Here's the drawing with two shaded views (mm, measured from the low corner). I have some questions. Coordinates: 2 decimals unless noted, no trailing zeros. Loops run counter-clockwise (first coordinate to the right, second up) from the corner with the lowest first, then second, coordinate; pieces in that order, holes last.
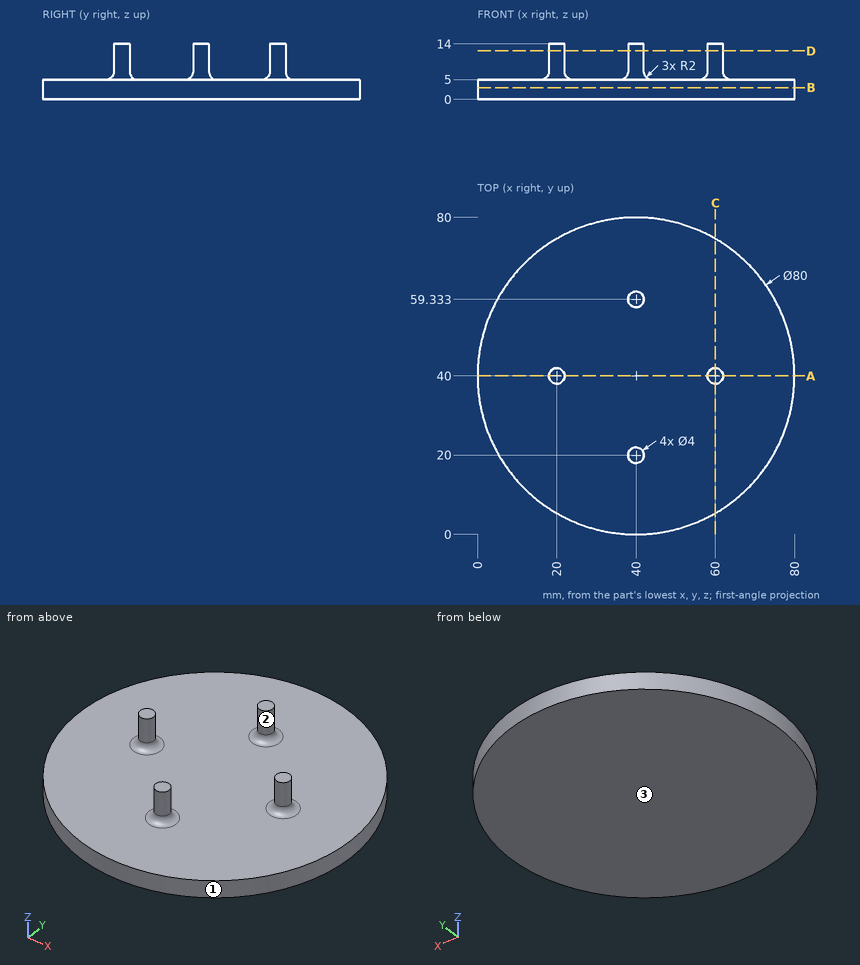
(1) I'm going to push flat-ended pins straight in: pin 1 (4 mm diameter, centred on x = 65.5, y = 39, fed in from -Z); pin 2 (5 mm diameter, centred on x = 53, y = 18, fed in from +Z); pin 3 (6 mm diameter, centred on y = 36, z = 2, fed in from -X); pin 4 (2 mm diameter, centred on x = 32.5, z = 4, fed in from -Y). Where does each tip first touch, or does it pass through?
Check values:
pin 1: stops at z = 0
pin 2: stops at z = 5
pin 3: stops at x = 0.01
pin 4: stops at y = 0.53
(2) If we mould it in two halves opening along Y, with no side actions, what happens to the marked faces 1, 2 and 3? For each: released by +Y, released by -Y, zero draft, split by the parting line, or undercut.
Check values:
face 1: split by the parting line
face 2: undercut
face 3: zero draft
(3) I want a section at A-A on y = 40. Write out the boundary of the cut face in (x, z).
Check values:
outline: (0, 0) - (80, 0) - (80, 5) - (64, 5) arc R2 cw to (62, 7) - (62, 14) - (58, 14) - (58, 7) arc R2 cw to (56, 5) - (24, 5) arc R2 cw to (22, 7) - (22, 14) - (18, 14) - (18, 7) arc R2 cw to (16, 5) - (0, 5) - close
(4) I want a section at B-B on z = 3. Write out the boundary of the cut face in (x, y), then the cut area to 3 significant figures.
Check values:
outline: circle Ø80 at (40, 40)
area: 5,030 mm2
(5) If I drill on probe 1 along Z at (x, y) = (26, 76); probe 2 along Y at (x, z) = (61, 7.25); probe 3 along X at (y, z) = (59.5, 6), over which ranges is the centre line in solid material (lowest first)?
Check values:
probe 1: z = 0 to 5
probe 2: y = 38.27 to 41.73
probe 3: x = 37.74 to 42.26
(6) I want a section at C-C on x = 60. Write out the boundary of the cut face in (y, z), then the cut area to 3 significant figures.
Check values:
outline: (5.36, 0) - (74.64, 0) - (74.64, 5) - (44, 5) arc R2 cw to (42, 7) - (42, 14) - (38, 14) - (38, 7) arc R2 cw to (36, 5) - (5.36, 5) - close
area: 384 mm2
(7) I want a section at D-D on z = 12.25. Write out the boundary of the cut face in (x, y).
Check values:
outline: circle Ø4 at (20, 40); circle Ø4 at (40, 20); circle Ø4 at (40, 59.33); circle Ø4 at (60, 40)
